from build123d import *

# Parameters (mm, degrees)
F0_W     = 160.1724
F0_H     = 301.371
F1_DEPTH = 3.175
F2_W     = 158.75
F2_H     = 40.64
F2_H_2   = 51.562
F2_H_3   = 38.1
F2_H_4   = 41.402
F3_DEPTH = 0.762


with BuildPart() as f1:
    # F0 (on Front) → F1 (new body)
    with BuildSketch(Plane.XZ):
        with Locations((580.1487, 150.6855)):
            Rectangle(F0_W, F0_H)
    extrude(amount=F1_DEPTH)

    # F2 (on face) → F3 (join)
    with BuildSketch(Plane.XZ.offset(3.175)):
        with Locations((580.1487, 281.051)):
            Rectangle(F2_W, F2_H)
        with Locations((580.1487, 182.88)):
            Rectangle(F2_W, F2_H_2)
        with Locations((580.1487, 103.251)):
            Rectangle(F2_W, F2_H_3)
        with Locations((580.1487, 20.701)):
            Rectangle(F2_W, F2_H_4)
    extrude(amount=F3_DEPTH)


solid = f1.part
Design review of the part built by this model. Coordinates are the model's own, in mm. Coordinates: 2 decimals unless noted, no trailing zeros. Loops run counter-clockwise (first coordinate to the right, second up) from the corner with the lowest first, then second, coordinate; pieces in that order, holes last. Notation, with made-up numbers: (24, -2.5) -> (55, -2.5) arc R32 cw to (55, 25.5) -> close; hole circle Ø2 at (-15, -33.5). An arc over 180 degrees is marked (long way). Use a Markdown table: item, result. Add a question column.
Item 1: We need section A-A, the plane x = 621.5. Write out the cut boundary in (y, z) (3 decimals), and give its area (3 significant figures).
Item 2: The part is to be moulded in two halves that separate along Z. For faces 1 (the flat face through (579, -3.175, 153)), 2 (the flat face through (579, -3.937, 21)), say which applies: +Z half, -Z half, draft (parallel to the pull), parting line (faces both ways), or undercut.
Item 3: Wall thickness on L1, parallel to Z at x = 595, y = -3.25; L2, parallel to Y at x = 596.5, z = 223 (3 decimals); L3, parallel to X at y = -3.6, z = 106.5: over which ranges is each line inside the solid? List them lowest first. Write a range as from..to.
Item 4: We need section B-B, the plane z = 237. Write out the cut boundary in (x, y) (1 decimal).
Item 5: Clearance check with flat-ended pins moving along their axes: P1, Ø0.8, axis at y = -3.5, z = 27.5, coming from the -X side; P2, Ø1.5, axis at x = 556.5, z = 64, coming from the -Y side (3 decimals). State where each tip first meets the part, or that it passes through.
Numbers:
| question | item | result |
|---|---|---|
| 1 | outline | (-3.937, 0) -> (0, 0) -> (0, 301.371) -> (-3.937, 301.371) -> (-3.937, 260.731) -> (-3.175, 260.731) -> (-3.175, 208.661) -> (-3.937, 208.661) -> (-3.937, 157.099) -> (-3.175, 157.099) -> (-3.175, 122.301) -> (-3.937, 122.301) -> (-3.937, 84.201) -> (-3.175, 84.201) -> (-3.175, 41.402) -> (-3.937, 41.402) -> close |
| 1 | area | 1,090 mm^2 |
| 2 | face 1 | undercut |
| 2 | face 2 | draft |
| 3 | L1 | z = 0..41.4, 84.2..122.3, 157.1..208.66, 260.73..301.37 |
| 3 | L2 | y = -3.175..0 |
| 3 | L3 | x = 500.77..659.52 |
| 4 | outline | (500.1, -3.2) -> (660.2, -3.2) -> (660.2, 0) -> (500.1, 0) -> close |
| 5 | P1 | stops at x = 500.06 |
| 5 | P2 | stops at y = -3.175 |
